The listing builds one solid part. Answer for the finished solid, in the listing's coordinates (mm). Coordinates: 2 decimals unless noted, no trailing zeros. Order: outer loops, then holes, each group sorted by start corner. A loop starts at its lowest first (then second) coordinate and runs counter-clockwise, first axis right, second up. Notation, with made-up numbers: (-2, 20.5) - (6, 20.5) arc R29 ccw to (6, 43.5) - close; hole circle Ø7 at (84.25, 27). An arc over 180 degrees is marked (long way). Use a Markdown table: item, result. Add a question column.
Item 1: The part is cut by section B-B, the plane x = 0. Give the vertices of the cut face in (y, z) (3 decimals).
Item 2: The part is cut by section A-A, the plane z = 0. Give the vertices of the cut face in (x, y) (3 decimals).
Item 3: Flat-ended cylindrical pins translate along their axes: P1, Ø15, axis at x = 0, y = 898.525, coming from the +Z side (3 decimals); P2, Ø1.5, axis at y = 532, z = 12, coming from the -X side; P3, Ø5, axis at y = -574.5, z = 12.5, coming from the +X side. Find the tip coordinate at first contact, or state that the pin passes through.
Item 4: Find the intervals of material crossed by line 1 along Z through (x, y) = (5, 431.5) (3 decimals); line 2 along Y through (x, z) = (0, -13.95), in increasing order.
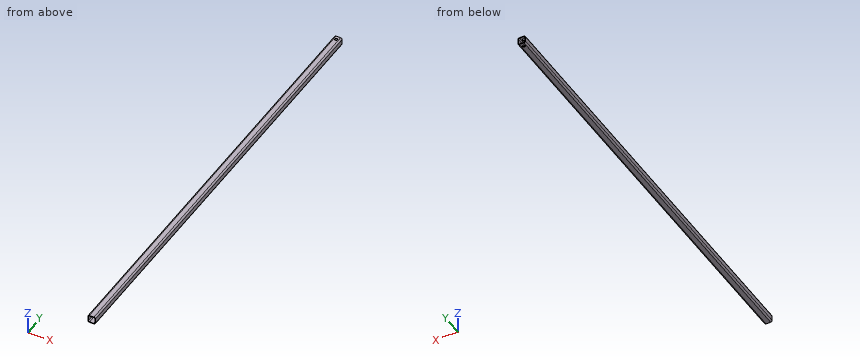
from build123d import *

# Parameters (mm, degrees)
BOSS_EXTRUDE1_DEPTH = 914.4
SKETCH2_R           = 5.715
CUT_EXTRUDE1_DEPTH  = 32.75


with BuildPart() as part:
    # Sketch1 → Boss-Extrude1 (new body, symmetric)
    with BuildSketch(Plane(origin=(0, 0, 0), x_dir=(1, 0, 0), z_dir=(0, 1, 0))):
        with BuildLine():
            Line((-9.525, -15.875), (9.525, -15.875))
            ThreePointArc((9.525, -15.875), (14.015128061, -14.015128061), (15.875, -9.525))
            Line((15.875, -9.525), (15.875, 9.525))
            ThreePointArc((15.875, 9.525), (14.015128061, 14.015128061), (9.525, 15.875))
            Line((9.525, 15.875), (-9.525, 15.875))
            ThreePointArc((-9.525, 15.875), (-14.015128061, 14.015128061), (-15.875, 9.525))
            Line((-15.875, 9.525), (-15.875, -9.525))
            ThreePointArc((-15.875, -9.525), (-14.015128061, -14.015128061), (-9.525, -15.875))
        make_face()
        with BuildLine():
            Line((-8.6995, -13.462), (8.6995, -13.462))
            ThreePointArc((8.6995, -13.462), (12.067096045, -12.067096045), (13.462, -8.6995))
            Line((13.462, -8.6995), (13.462, 8.6995))
            ThreePointArc((13.462, 8.6995), (12.067096045, 12.067096045), (8.6995, 13.462))
            Line((8.6995, 13.462), (-8.6995, 13.462))
            ThreePointArc((-8.6995, 13.462), (-12.067096045, 12.067096045), (-13.462, 8.6995))
            Line((-13.462, 8.6995), (-13.462, -8.6995))
            ThreePointArc((-13.462, -8.6995), (-12.067096045, -12.067096045), (-8.6995, -13.462))
        make_face(mode=Mode.SUBTRACT)
    extrude(amount=BOSS_EXTRUDE1_DEPTH, both=True)

    # Sketch2 → Cut-Extrude1 (cut, through all)
    with BuildSketch(Plane.XY.offset(15.875)):
        with Locations((0, 898.525)):
            Circle(SKETCH2_R)
    extrude(amount=-CUT_EXTRUDE1_DEPTH, mode=Mode.SUBTRACT)


solid = part.part
Solution:
| question | item | result |
|---|---|---|
| 1 | outline | (-914.4, -15.875) - (892.81, -15.875) - (892.81, -13.462) - (-914.4, -13.462) - close; (-914.4, 13.462) - (892.81, 13.462) - (892.81, 15.875) - (-914.4, 15.875) - close; (904.24, -15.875) - (914.4, -15.875) - (914.4, -13.462) - (904.24, -13.462) - close; (904.24, 13.462) - (914.4, 13.462) - (914.4, 15.875) - (904.24, 15.875) - close |
| 2 | outline | (-15.875, -914.4) - (-13.462, -914.4) - (-13.462, 914.4) - (-15.875, 914.4) - close; (13.462, -914.4) - (15.875, -914.4) - (15.875, 914.4) - (13.462, 914.4) - close |
| 3 | P1 | stops at z = 15.875 |
| 3 | P2 | stops at x = -15.64 |
| 3 | P3 | stops at x = 15.86 |
| 4 | line 1 | z = -15.875 to -13.462, 13.462 to 15.875 |
| 4 | line 2 | y = -914.4 to 892.81, 904.24 to 914.4 |
